Build history of the part. All positions in model axes, mm. A direction names the side the tool comes from. Round coordinates to 2 decimals unless told otherwise and drop trailing zeros. Write each loop counter-clockwise with the first axis right and the second up, starting at its lowest first coordinate (ties: lowest second). Pieces come first, ordered by that corner, then holes. Notation, with made-up numbers: M -20.5,54 L 29.5,54 A27 cw 29.5,82 Z; hole C 28.5,-6.75 d5. An arc over 180 degrees is marked long. Write item = value, one per line. Start each with the question number.
Q1. Band-saw the part on C-C on y = 1. Write the cut outline in (x, z), plus the area to 3 significant figures.
Q2. Band-saw the part on B-B on x = -9.5. Write the cut outline in (y, z), plus the area to 3 significant figures.
Q3. Band-saw the part on A-A on z = 0. State how many separate pieces and enclosed holes the cut face has, plus the area to 3 significant figures.
Q4. Tool access for faces 4 (the flat face through (-11, 0, 0)), 5 (the flat face through (0, -3, -3.7)): list every direction of +Z, -Z, +X, -X, +Y, -Y with a clear straight run to the whole face (end or side of a thin tool).
Q5. Probe L1, parallel to X at y = -2.25, z = 1.25; L2, parallel to Y at x = 7, z = -3.25; L3, parallel to Y at x = 9.75, z = 1.75. List the from-to ranges inside material, lowest first.
Q6. Pull direction Z, two halves, no side cores. Call faces 1 (the flat face through (7.75, -3, 0)), 2 (the flat face through (2, 0, 0)), 3 (the cylindrical face through (11.349, 0.246, 2.815)): released by +Z, released by -Z, zero draft, split by the parting line, or undercut.
Q7. Band-saw the part on D-D on z = -2.5. Write the cut outline in (x, y).
Q8. Drop flat-ended pins along their axis: P1, Ø1, axis at x = -2.5, z = 3, coming from the -Y side; P2, Ø2, axis at x = -3.5, y = -8, coming from the +Z side; P3, Ø1.1, axis at y = 3, z = 0, coming from the -X side. Give the stop position or say it passes through.
```python
from build123d import *

# Parameters (mm, degrees)
CROQUIS1_R              = 1
SALIENTE_EXTRUIR1_DEPTH = 0.5
CROQUIS2_W              = 15.5
CROQUIS2_H              = 7.4
SALIENTE_EXTRUIR2_DEPTH = 6.7
CROQUIS3_W              = 1.8
CROQUIS3_H              = 0.46
SALIENTE_EXTRUIR3_DEPTH = 4.8
CROQUIS4_W              = 8.8
CROQUIS4_H              = 4.2
CORTAR_EXTRUIR1_DEPTH   = 0.5
CROQUIS5_W              = 5.5
CROQUIS5_H              = 3.8
SALIENTE_EXTRUIR4_DEPTH = 5
CORTAR_EXTRUIR2_REACH   = 19.185
CROQUIS6_RX             = 0.9
CROQUIS6_RY             = 0.55
REDONDEO2_R             = 0.5
CORTAR_EXTRUIR3_REACH   = 19.301


with BuildPart() as part:
    # Croquis1 → Saliente-Extruir1 (new body)
    with BuildSketch(Plane(origin=(0, 0, 0), x_dir=(1, 0, 0), z_dir=(0, 1, 0))):
        with BuildLine():
            Line((10.65, 3.1), (7.75, 3.1))
            Line((7.75, 3.1), (7.75, 3.7))
            Line((7.75, 3.7), (-7.75, 3.7))
            Line((-7.75, 3.7), (-7.75, 3.1))
            Line((-7.75, 3.1), (-10.65, 3.1))
            ThreePointArc((-10.65, 3.1), (-11.357106781, 2.807106781), (-11.65, 2.1))
            Line((-11.65, 2.1), (-11.65, -2.1))
            ThreePointArc((-11.65, -2.1), (-11.357106781, -2.807106781), (-10.65, -3.1))
            Line((-10.65, -3.1), (-7.75, -3.1))
            Line((-7.75, -3.1), (-7.75, -3.7))
            Line((-7.75, -3.7), (7.75, -3.7))
            Line((7.75, -3.7), (7.75, -3.1))
            Line((7.75, -3.1), (10.65, -3.1))
            ThreePointArc((10.65, -3.1), (11.357106781, -2.807106781), (11.65, -2.1))
            Line((11.65, -2.1), (11.65, 2.1))
            ThreePointArc((11.65, 2.1), (11.357106781, 2.807106781), (10.65, 3.1))
        make_face()
        with Locations(Location((9.5, 0, 0), (0, 0, 270))):
            Circle(CROQUIS1_R, mode=Mode.SUBTRACT)
        with Locations(Location((-9.5, 0, 0), (0, 0, 270))):
            Circle(CROQUIS1_R, mode=Mode.SUBTRACT)
    extrude(amount=SALIENTE_EXTRUIR1_DEPTH)

    # Croquis2 → Saliente-Extruir2 (add)
    with BuildSketch(Plane.XZ):
        Rectangle(CROQUIS2_W, CROQUIS2_H)
    extrude(amount=SALIENTE_EXTRUIR2_DEPTH)

    # Croquis3 → Saliente-Extruir3 (add)
    with BuildSketch(Plane.XZ.offset(6.7)):
        with Locations((0, -1.3)):
            Rectangle(CROQUIS3_W, CROQUIS3_H)
        with Locations((-4, -1.3)):
            Rectangle(CROQUIS3_W, CROQUIS3_H)
        with Locations((4, -1.3)):
            Rectangle(CROQUIS3_W, CROQUIS3_H)
        with Locations((4, 1.3)):
            Rectangle(CROQUIS3_W, CROQUIS3_H)
        with Locations((-4, 1.3)):
            Rectangle(CROQUIS3_W, CROQUIS3_H)
        with Locations((0, 1.3)):
            Rectangle(CROQUIS3_W, CROQUIS3_H)
    extrude(amount=SALIENTE_EXTRUIR3_DEPTH)

    # Croquis4 → Cortar-Extruir1 (cut)
    with BuildSketch(Plane(origin=(0, 0.5, 0), x_dir=(1, 0, 0), z_dir=(0, 1, 0))):
        Rectangle(CROQUIS4_W, CROQUIS4_H)
    extrude(amount=-CORTAR_EXTRUIR1_DEPTH, mode=Mode.SUBTRACT)

    # Croquis5 → Saliente-Extruir4 (add)
    with BuildSketch(Plane(origin=(0, 0, 0), x_dir=(1, 0, 0), z_dir=(0, 1, 0))):
        with Locations((-1.6, 0)):
            Rectangle(CROQUIS5_W, CROQUIS5_H)
    extrude(amount=SALIENTE_EXTRUIR4_DEPTH)

    # Cortar-Extruir2: up to this face of the body (flat: up to its plane)
    cortar_extruir2_end = Plane(part.part.faces().sort_by_distance((-4, -9.1, -1.53))[0])
    # Croquis6 → Cortar-Extruir2 (cut, up to the picked face)
    with BuildSketch(Plane.XY.offset(1.53), mode=Mode.PRIVATE) as cortar_extruir2_sk1:
        with Locations(Location((-4, -9.1), (0, 0, -90))):
            Ellipse(CROQUIS6_RX, CROQUIS6_RY)
    cortar_extruir2_tool1 = split(extrude(cortar_extruir2_sk1.sketch, amount=-CORTAR_EXTRUIR2_REACH, mode=Mode.PRIVATE), bisect_by=cortar_extruir2_end, keep=Keep.BOTH, mode=Mode.PRIVATE)
    # Croquis6 → Cortar-Extruir2 (cut, up to the picked face)
    with BuildSketch(Plane.XY.offset(1.53), mode=Mode.PRIVATE) as cortar_extruir2_sk2:
        with Locations(Location((0, -9.1), (0, 0, 90))):
            Ellipse(CROQUIS6_RX, CROQUIS6_RY)
    cortar_extruir2_tool2 = split(extrude(cortar_extruir2_sk2.sketch, amount=-CORTAR_EXTRUIR2_REACH, mode=Mode.PRIVATE), bisect_by=cortar_extruir2_end, keep=Keep.BOTH, mode=Mode.PRIVATE)
    # Croquis6 → Cortar-Extruir2 (cut, up to the picked face)
    with BuildSketch(Plane.XY.offset(1.53), mode=Mode.PRIVATE) as cortar_extruir2_sk3:
        with Locations(Location((4, -9.1), (0, 0, -90))):
            Ellipse(CROQUIS6_RX, CROQUIS6_RY)
    cortar_extruir2_tool3 = split(extrude(cortar_extruir2_sk3.sketch, amount=-CORTAR_EXTRUIR2_REACH, mode=Mode.PRIVATE), bisect_by=cortar_extruir2_end, keep=Keep.BOTH, mode=Mode.PRIVATE)
    add(cortar_extruir2_tool1.solids().sort_by(Axis((-4, -9.1, 1.53), (0, 0, -1)))[0], mode=Mode.SUBTRACT)
    add(cortar_extruir2_tool2.solids().sort_by(Axis((0, -9.1, 1.53), (0, 0, -1)))[0], mode=Mode.SUBTRACT)
    add(cortar_extruir2_tool3.solids().sort_by(Axis((4, -9.1, 1.53), (0, 0, -1)))[0], mode=Mode.SUBTRACT)

    # Redondeo2
    redondeo2_edges = [part.edges().sort_by_distance(p)[0] for p in [
        (0.9, -11.5, 1.3),
        (-0.9, -11.5, 1.3),
        (4.9, -11.5, 1.3),
        (3.1, -11.5, 1.3),
        (-3.1, -11.5, 1.3),
        (-4.9, -11.5, 1.3),
        (-0.9, -11.5, -1.3),
        (0.9, -11.5, -1.3),
        (-4.9, -11.5, -1.3),
        (-3.1, -11.5, -1.3),
        (3.1, -11.5, -1.3),
        (4.9, -11.5, -1.3),
    ]]
    fillet(redondeo2_edges, radius=REDONDEO2_R)

    # Croquis7 → Cortar-Extruir3 (cut, up to next)
    with BuildSketch(Plane.XY.offset(1.9), mode=Mode.PRIVATE) as cortar_extruir3_sk1:
        Polygon((-3.923177813, 5), (-4.35, 5), (-4.35, 4.573177813), align=None)
    cortar_extruir3_tool1 = extrude(cortar_extruir3_sk1.sketch, amount=-CORTAR_EXTRUIR3_REACH, mode=Mode.PRIVATE) & part.part
    # Croquis7 → Cortar-Extruir3 (cut, up to next)
    with BuildSketch(Plane.XY.offset(1.9), mode=Mode.PRIVATE) as cortar_extruir3_sk2:
        Polygon((1.15, 5), (0.460006212, 5), (1.15, 4.310006212), align=None)
    cortar_extruir3_tool2 = extrude(cortar_extruir3_sk2.sketch, amount=-CORTAR_EXTRUIR3_REACH, mode=Mode.PRIVATE) & part.part
    # Croquis7 → Cortar-Extruir3 (cut, up to next)
    with BuildSketch(Plane.XY.offset(1.9), mode=Mode.PRIVATE) as cortar_extruir3_sk3:
        Polygon((0.460006212, 5), (-0.699513597, 5), (-0.119753693, 4.420240095), align=None)
    cortar_extruir3_tool3 = extrude(cortar_extruir3_sk3.sketch, amount=-CORTAR_EXTRUIR3_REACH, mode=Mode.PRIVATE) & part.part
    # Croquis7 → Cortar-Extruir3 (cut, up to next)
    with BuildSketch(Plane.XY.offset(1.9), mode=Mode.PRIVATE) as cortar_extruir3_sk4:
        Polygon((-0.699513597, 5), (-1.824858034, 5), (-1.262185815, 4.437327782), align=None)
    cortar_extruir3_tool4 = extrude(cortar_extruir3_sk4.sketch, amount=-CORTAR_EXTRUIR3_REACH, mode=Mode.PRIVATE) & part.part
    # Croquis7 → Cortar-Extruir3 (cut, up to next)
    with BuildSketch(Plane.XY.offset(1.9), mode=Mode.PRIVATE) as cortar_extruir3_sk5:
        Polygon((-1.824858034, 5), (-2.880534962, 5), (-2.352696498, 4.472161536), align=None)
    cortar_extruir3_tool5 = extrude(cortar_extruir3_sk5.sketch, amount=-CORTAR_EXTRUIR3_REACH, mode=Mode.PRIVATE) & part.part
    # Croquis7 → Cortar-Extruir3 (cut, up to next)
    with BuildSketch(Plane.XY.offset(1.9), mode=Mode.PRIVATE) as cortar_extruir3_sk6:
        Polygon((-2.880534962, 5), (-3.923177813, 5), (-3.401856388, 4.478678575), align=None)
    cortar_extruir3_tool6 = extrude(cortar_extruir3_sk6.sketch, amount=-CORTAR_EXTRUIR3_REACH, mode=Mode.PRIVATE) & part.part
    add(cortar_extruir3_tool1.solids().sort_by_distance((-4.207726, 4.857726, 1.9))[0], mode=Mode.SUBTRACT)
    add(cortar_extruir3_tool2.solids().sort_by_distance((0.920002, 4.770002, 1.9))[0], mode=Mode.SUBTRACT)
    add(cortar_extruir3_tool3.solids().sort_by_distance((-0.119754, 4.806747, 1.9))[0], mode=Mode.SUBTRACT)
    add(cortar_extruir3_tool4.solids().sort_by_distance((-1.262186, 4.812443, 1.9))[0], mode=Mode.SUBTRACT)
    add(cortar_extruir3_tool5.solids().sort_by_distance((-2.352696, 4.824054, 1.9))[0], mode=Mode.SUBTRACT)
    add(cortar_extruir3_tool6.solids().sort_by_distance((-3.401856, 4.826226, 1.9))[0], mode=Mode.SUBTRACT)


solid = part.part
```
Conclusion:
q1.outline = M -4.35,-1.9 L 1.15,-1.9 L 1.15,1.9 L -4.35,1.9 Z
q1.area = 20.9 mm^2
q2.outline = M 0,-3.1 L 0.5,-3.1 L 0.5,-1 L 0,-1 Z; M 0,1 L 0.5,1 L 0.5,3.1 L 0,3.1 Z
q2.area = 2.10 mm^2
q3.separate_pieces = 3
q3.enclosed_holes = 0
q3.area = 135 mm^2
q4.face_4 = +Z, -Z, -X, -Y
q4.face_5 = -Z, +X, -X, +Y, -Y
q5.L1 = -7.75 to 7.75
q5.L2 = -6.7 to 0.5
q5.L3 = 0 to 0.5
q6.face_1 = zero draft
q6.face_2 = undercut
q6.face_3 = released by +Z
q7.outline = M -11.57,0 L -7.75,0 L -7.75,-6.7 L 7.75,-6.7 L 7.75,0 L 11.57,0 L 11.57,0.5 L -11.57,0.5 Z
q8.P1 = -6.7
q8.P2 = 1.53
q8.P3 = -4.35
